Could you check a few things on this model? Use its own coordinates, in mm. Face numbers are marked on the shaded views. A direction names the side the tool comes from. Round coordinates to 2 decimals unless told otherwise and drop trailing zeros. Loops run counter-clockwise (first coordinate to the right, second up) from the corner with the lowest first, then second, coordinate; pieces in that order, holes last. Notation, with made-up numbers: (-24, 50) -> (-2, 50) arc R23 cw to (-2, 67) -> close; hole circle Ø3 at (15.5, 69.5). An arc over 180 degrees is marked (long way). Write each question's results on one line, items separated by ' | '. Start each with the question number.
1) Which directions (+Z, -Z, +X, -X, +Y, -Y) give clear straight access to the entire face, cutting with the end or side of a thin tool? Please do the marked faces 1, 2 and 3.
2) Imagine slicing it at B-B, the plane z = -1311. List the corners of the cut face in (x, y) for me, plus the area to 3 significant figures.
3) Imagine slicing it at A-A, the plane x = 1506.5. List the corners of the cut face in (y, z) for me, plus the area to 3 significant figures.
4) For P1, Ø5, axis at x = 1028.5, y = 267.5, coming from the +Z side; P2, Ø3, axis at x = 869, y = 314, coming from the -Z side, each with a flat end and sliding along its axis, tell me the tip position at first contact or that it passes through.
5) Imagine slicing it at C-C, the plane y = 444.5. List the corners of the cut face in (x, z) for me, plus the area to 3 significant figures.
6) If I drill on probe 1 along Y at (x, z) = (1628, 102.5); probe 2 along Z at (x, y) = (1371, 185), over which ranges is the centre line in solid material (lowest first)?
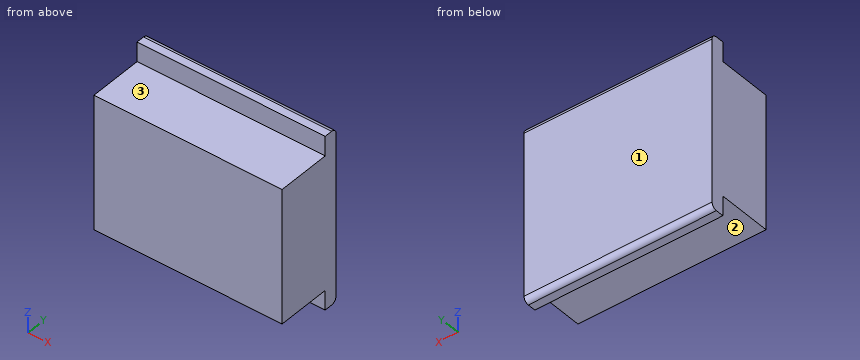
from build123d import *

# Parameters (mm, degrees)
BOSS_EXTRUDE1_DEPTH = 1778


with BuildPart() as part:
    # Sketch1 → Boss-Extrude1 (new body)
    with BuildSketch(Plane(origin=(0, 0, 0), x_dir=(0, 0, -1), z_dir=(1, 0, 0))):
        with BuildLine():
            Line((0, 0), (1270, 0))
            Line((1270, 0), (1270, 508))
            Line((1270, 508), (1455.096882898, 508))
            Line((1455.096882898, 508), (1455.096882898, 584.2))
            ThreePointArc((1455.096882898, 584.2), (1440.217907382, 620.121024484), (1404.296882898, 635))
            Line((1404.296882898, 635), (-134.296882898, 635))
            ThreePointArc((-134.296882898, 635), (-170.217907382, 620.121024484), (-185.096882898, 584.2))
            Line((-185.096882898, 584.2), (-185.096882898, 508))
            Line((-185.096882898, 508), (0, 508))
            Line((0, 508), (0, 0))
        make_face()
    extrude(amount=BOSS_EXTRUDE1_DEPTH)


solid = part.part
Checked values:
1) face 1: +Z, -Z, +X, -X, +Y | face 2: -Z, +X, -X, -Y | face 3: +Z, +X, -X, -Y
2) outline: (0, 508) -> (1778, 508) -> (1778, 635) -> (0, 635) -> close | area: 226,000 mm^2
3) outline: (0, -1270) -> (508, -1270) -> (508, -1455.1) -> (584.2, -1455.1) arc R50.8 ccw to (635, -1404.3) -> (635, 134.3) arc R50.8 ccw to (584.2, 185.1) -> (508, 185.1) -> (508, 0) -> (0, 0) -> close | area: 852,000 mm^2
4) P1: z = 0 | P2: z = -1270
5) outline: (0, -1270) -> (1778, -1270) -> (1778, 0) -> (0, 0) -> close | area: 2,260,000 mm^2
6) probe 1: 508 to 635 | probe 2: -1270 to 0
